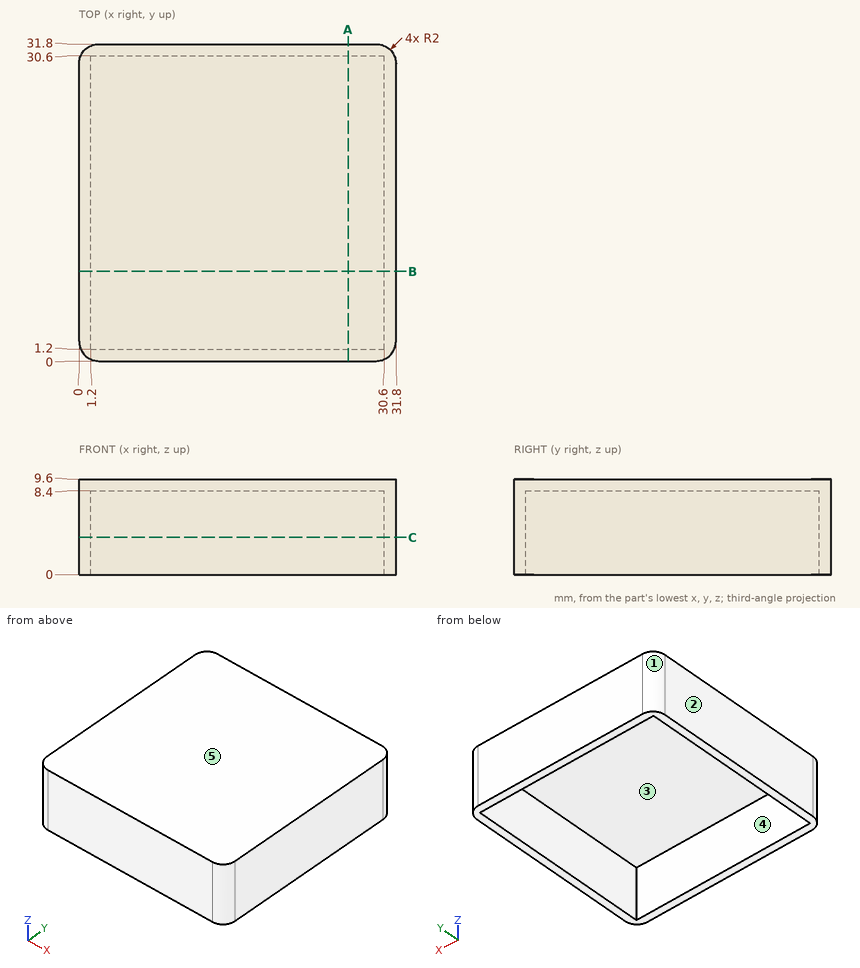
Check sheet for the drawn part. Datum: minimum x, y, z corner. Units: mm. A direction names the side the tool comes from. Coordinates: 2 decimals unless noted, no trailing zeros. Loops run counter-clockwise (first coordinate to the right, second up) from the corner with the lowest first, then second, coordinate; pieces in that order, holes last. Notation, with made-up numbers: (-30.75, 34) -> (-15.75, 34) arc R8 cw to (-15.75, 39) -> close; hole circle Ø3 at (6, -32). An arc over 180 degrees is marked (long way). Write each question's results on one line, items separated by ' | '.
Item 1: Mould release check, pull along Y, two halves, no side actions. Record for the marked faces 1, 2 and 3: +Y half, -Y half, draft (parallel to the pull), parting line (faces both ways), or undercut.
Found:
face 1: +Y half | face 2: draft | face 3: undercut
Item 2: Material ranges on L1, parallel to Y at x = 3, z = 2.5; L2, parallel to Z at x = 10, y = 30, recorded low to high.
Found:
L1: y = 0 to 1.2, 30.6 to 31.8 | L2: z = 8.4 to 9.6
Item 3: Section check C-C, the plane z = 3.75. Enter the section's corners in (x, y).
Found:
outline: (0, 2) arc R2 ccw to (2, 0) -> (29.8, 0) arc R2 ccw to (31.8, 2) -> (31.8, 29.8) arc R2 ccw to (29.8, 31.8) -> (2, 31.8) arc R2 ccw to (0, 29.8) -> close; hole (1.2, 1.2) -> (30.6, 1.2) -> (30.6, 30.6) -> (1.2, 30.6) -> close
Item 4: Tool access check on the marked faces 4 and 5. Record the directions out of +Z, -Z, +X, -X, +Y, -Y that give a thin tool (end or side, any length) a straight path to the whole face; none if there is none.
Found:
face 4: -Z | face 5: +Z, +X, -X, +Y, -Y
Item 5: Section check A-A, the plane x = 27. Enter the section's corners in (y, z), plus the area to 3 significant figures.
Found:
outline: (0, 0) -> (1.2, 0) -> (1.2, 8.4) -> (30.6, 8.4) -> (30.6, 0) -> (31.8, 0) -> (31.8, 9.6) -> (0, 9.6) -> close | area: 58.3 mm2
Item 6: Gauge pin test, flat end, axial feed: pin 1 (1.5 mm diameter, centred on x = 25.5, z = 2.5, fed in from -Y). Record the tip position at first contact, or that the pin passes through.
Found:
pin 1: stops at y = 0
